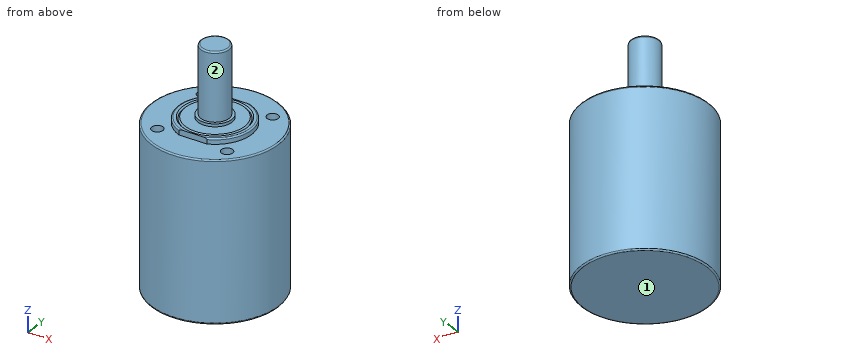
```python
from build123d import *

# Parameters (mm, degrees)
FILLET1_R          = 0.5
CUT_EXTRUDE1_DEPTH = 2
SKETCH4_R          = 2
CUT_EXTRUDE2_DEPTH = 8


with BuildPart() as part:
    # Sketch1 → Revolve1 (revolve)
    with BuildSketch(Plane(origin=(0, 0, 0), x_dir=(0, 0, -1), z_dir=(1, 0, 0))):
        Polygon((0, 0), (0, 22.5), (-56.2, 22.5), (-56.2, 13), (-58.2, 13), (-58.2, 11.5), (-57.7, 11), (-58.2, 10.5), (-58.2, 6), (-59.2, 6), (-59.2, 5), (-83.2, 5), (-83.2, 0), align=None)
    revolve(axis=Axis((0, 0, 0), (0, 0, 1)))

    # Fillet1
    fillet1_edges = [part.edges().sort_by_distance(p)[0] for p in [
        (0, -5, 83.2),
        (0, -13, 58.2),
        (0, -22.5, 56.2),
        (0, -22.5, 0),
    ]]
    fillet(fillet1_edges, radius=FILLET1_R)

    # Sketch3 → Cut-Extrude1 (cut)
    with BuildSketch(Plane.XY.offset(58.2)):
        with BuildLine():
            Line((-5, 12), (5, 12))
            ThreePointArc((5, 12), (0, 13), (-5, 12))
        make_face()
        with BuildLine():
            Line((-5, -12), (5, -12))
            ThreePointArc((5, -12), (0, -13), (-5, -12))
        make_face()
    extrude(amount=-CUT_EXTRUDE1_DEPTH, mode=Mode.SUBTRACT)

    # Sketch4 → Cut-Extrude2 (cut)
    with BuildSketch(Plane.XY.offset(56.2)):
        with Locations((-12.374368671, 12.374368671)):
            Circle(SKETCH4_R)
        with Locations((12.374368671, 12.374368671)):
            Circle(SKETCH4_R)
        with Locations((12.374368671, -12.374368671)):
            Circle(SKETCH4_R)
        with Locations((-12.374368671, -12.374368671)):
            Circle(SKETCH4_R)
    extrude(amount=-CUT_EXTRUDE2_DEPTH, mode=Mode.SUBTRACT)


solid = part.part
```
For this review, take the finished solid that the model builds, in its own axes (mm). Face numbers are marked on the shaded views. A direction names the side the tool comes from. Round coordinates to 2 decimals unless told otherwise and drop trailing zeros. Order: outer loops, then holes, each group sorted by start corner. A loop starts at its lowest first (then second) coordinate and runs counter-clockwise, first axis right, second up. Notation, with made-up numbers: (23.25, 66.5) -> (64.25, 66.5) arc R21 cw to (64.25, 81.5) -> close; hole circle Ø11 at (10.25, 44). An arc over 180 degrees is marked (long way). Use a Markdown table: item, result.
Item 1: Take a section at B-B (x = 0). State the section outline as (y, z) points, plus the area to 3 significant figures.
Resolved:
| item | result |
|---|---|
| outline | (-22.5, 0.5) arc R0.5 ccw to (-22, 0) -> (22, 0) arc R0.5 ccw to (22.5, 0.5) -> (22.5, 55.7) arc R0.5 ccw to (22, 56.2) -> (12, 56.2) -> (12, 58.2) -> (11.5, 58.2) -> (11, 57.7) -> (10.5, 58.2) -> (6, 58.2) -> (6, 59.2) -> (5, 59.2) -> (5, 82.7) arc R0.5 ccw to (4.5, 83.2) -> (-4.5, 83.2) arc R0.5 ccw to (-5, 82.7) -> (-5, 59.2) -> (-6, 59.2) -> (-6, 58.2) -> (-10.5, 58.2) -> (-11, 57.7) -> (-11.5, 58.2) -> (-12, 58.2) -> (-12, 56.2) -> (-22, 56.2) arc R0.5 ccw to (-22.5, 55.7) -> close |
| area | 2,830 mm² |
Item 2: Take a section at D-D (z = 16). State the section outline as (x, y) points, plus the area to 3 significant figures.
Resolved:
| item | result |
|---|---|
| outline | circle Ø45 at (0, 0) |
| area | 1,590 mm² |
Item 3: Take a section at C-C (z = 49.5). State the section outline as (x, y) points, plus the area to 3 significant figures.
Resolved:
| item | result |
|---|---|
| outline | circle Ø45 at (0, 0); hole circle Ø4 at (-12.37, -12.37); hole circle Ø4 at (-12.37, 12.37); hole circle Ø4 at (12.37, -12.37); hole circle Ø4 at (12.37, 12.37) |
| area | 1,540 mm² |
Item 4: For line 1 along Z through (x, y) = (-15.5, 0.5); line 2 along Z through (x, y) = (11, -5); line 3 along X through (y, z) = (0, 35), list the stretches that pass through material, from the lowest coordinate up. Write a range as [from, to].
Resolved:
| item | result |
|---|---|
| line 1 | z = [0, 56.2] |
| line 2 | z = [0, 58.2] |
| line 3 | x = [-22.5, 22.5] |
Item 5: For pin 1 (1.5 mm diameter, centred on x = 7, y = 13.5, fed in from +Z); pin 2 (12 mm diameter, centred on y = -5.5, z = 29.5, fed in from +X); pin 3 (2 mm diameter, centred on x = -3, z = 29.5, fed in from -Y), all flat-tipped, find the tip position at first contact; note any pin that passes through.
Resolved:
| item | result |
|---|---|
| pin 1 | stops at z = 56.2 |
| pin 2 | stops at x = 22.5 |
| pin 3 | stops at y = -22.41 |
Item 6: Machinability: for the marked faces 1 and 2, which of the approach directions +Z, -Z, +X, -X, +Y, -Y give a long, thin tool a straight path to every point of the face, cutting with its end or side? Answer none if there is none.
Resolved:
| item | result |
|---|---|
| face 1 | -Z, +X, -X, +Y, -Y |
| face 2 | +Z |
